```python
from build123d import *

# Parameters (mm, degrees)
SKETCH1_R             = 4.7625
BOSS_EXTRUDE1_DEPTH   = 19.05
CHAMFER1_SIZE         = 1.016
CHAMFER1_SIZE2        = 0.883195326
CHAMFER1_PART_2_SIZE  = 1.016
CHAMFER1_PART_2_SIZE2 = 0.883195326


with BuildPart() as part:
    # Sketch1 → Boss-Extrude1 (new body, symmetric)
    with BuildSketch(Plane(origin=(0, 0, 0), x_dir=(1, 0, 0), z_dir=(0, 1, 0))):
        Circle(SKETCH1_R)
    extrude(amount=BOSS_EXTRUDE1_DEPTH, both=True)

    # Chamfer1
    chamfer1_edges = [part.edges().sort_by_distance(p)[0] for p in [
        (-4.7625, -19.05, 0),
    ]]
    chamfer1_side = [part.faces().sort_by_distance(p)[0] for p in [
        (0, -19.05, 0),
    ]]
    chamfer(chamfer1_edges, length=CHAMFER1_SIZE, length2=CHAMFER1_SIZE2, reference=chamfer1_side[0])

    # Chamfer1 part 2
    chamfer1_part_2_edges = [part.edges().sort_by_distance(p)[0] for p in [
        (-4.7625, 19.05, 0),
    ]]
    chamfer1_part_2_side = [part.faces().sort_by_distance(p)[0] for p in [
        (-4.7625, 0, 0),
    ]]
    chamfer(chamfer1_part_2_edges, length=CHAMFER1_PART_2_SIZE, length2=CHAMFER1_PART_2_SIZE2, reference=chamfer1_part_2_side[0])


solid = part.part
```
Build history of the part. All positions in model axes, mm. Give positions to 0.01 mm unless a question says otherwise; leave off trailing zeros. Loops run counter-clockwise (first coordinate to the right, second up) from the corner with the lowest first, then second, coordinate; pieces in that order, holes last.
1) Band-saw the part on A-A on y = 12.5. List the corners of the cut face in (x, z) (1 decimal), then the cut area to 3 significant figures.
Values follow:
outline: circle Ø9.5 at (0, 0)
area: 71.3 mm2
2) Drop flat-ended pins along their axis: P1, Ø4, axis at x = -3, z = -3, coming from the -Y side; P2, Ø5, axis at y = 15, z = 3.5, coming from the -X side; P3, Ø4, axis at x = 3.5, y = -9.5, coming from the +Z side. Give the stop position or say it passes through.
Values follow:
P1: stops at y = -19.05
P2: stops at x = -4.66
P3: stops at z = 4.52
3) Probe line 1 along X through (y, z) = (-16, -0.25); line 2 along Z through (x, y) = (-2.75, 12.5). List the from-to ranges inside material, lowest first.
Values follow:
line 1: x = -4.76 to 4.76
line 2: z = -3.89 to 3.89
